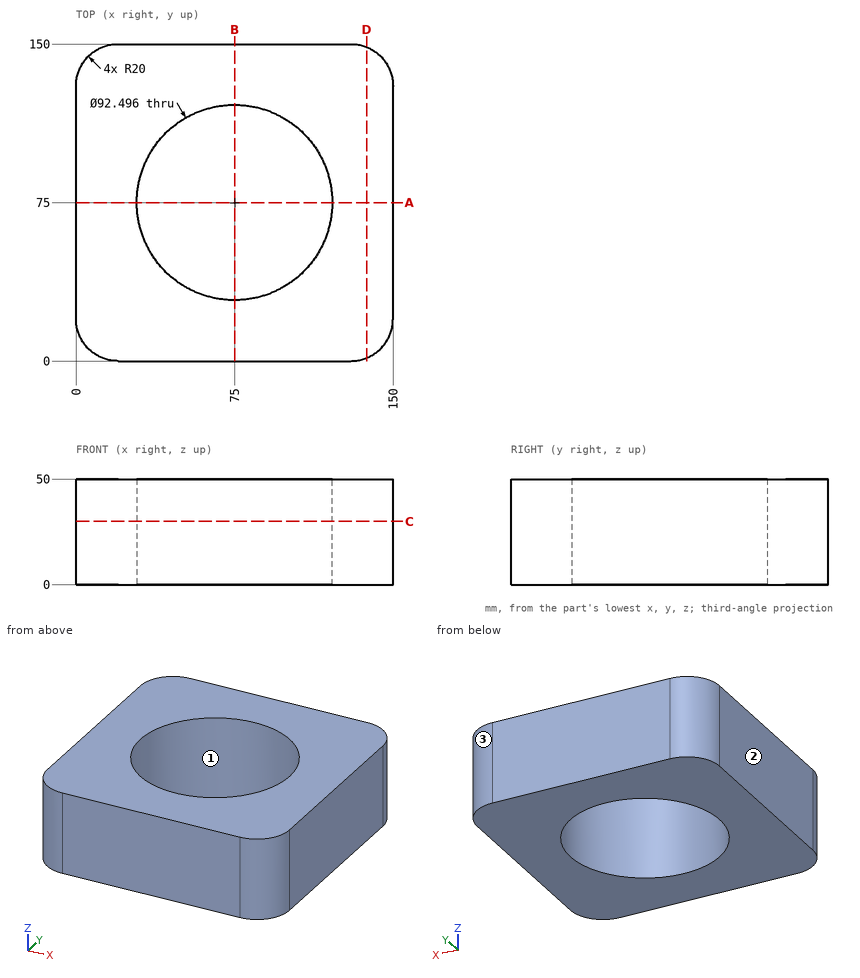
Print and shaded views of the part. All mm, measured from the part's lowest x, y and z. Give positions to 0.01 mm unless a question says otherwise; leave off trailing zeros. Write each loop counter-clockwise with the first axis right and the second up, starting at its lowest first coordinate (ties: lowest second). Pieces come first, ordered by that corner, then holes. Notation, with made-up numbers: (2, -19) -> (20, -19) arc R15 ccw to (20, -4) -> close; hole circle Ø7 at (11.5, 10.25). An arc over 180 degrees is marked (long way). Use CSV: the item, a comma, the result in double quotes. Start each with the question number.
1) Cut at C-C on z = 30. List the corners of the cut face in (x, y), plus the area to 3 significant figures.
2) Drill centre lines: L1, parallel to X at y = 75, z = 38.5; L2, parallel to X at y = 38.5, z = 36.5. Where is each one in solid material? Low to high.
3) Cut at D-D on x = 137.5. List the corners of the cut face in (y, z).
4) Pin check, flat tip, straight feed: P1, Ø5, axis at y = 18, z = 31, coming from the -X side. Stop position of the tip, or through.
5) Cut at A-A on y = 75. List the corners of the cut face in (x, z).
6) Two-plate mould, pull along Y, no slides. Class the marked faces 1, 2 and 3: released by +Y, released by -Y, zero draft, split by the parting line, or undercut.
Final values:
1,outline,"(0, 20) arc R20 ccw to (20, 0) -> (130, 0) arc R20 ccw to (150, 20) -> (150, 130) arc R20 ccw to (130, 150) -> (20, 150) arc R20 ccw to (0, 130) -> close; hole circle Ø92.5 at (75, 75)"
1,area,"15,400 mm2"
2,L1,"x = 0 to 28.75, 121.25 to 150"
2,L2,"x = 0 to 46.6, 103.4 to 150"
3,outline,"(1.46, 0) -> (148.54, 0) -> (148.54, 50) -> (1.46, 50) -> close"
4,P1,"stops at x = 0"
5,outline,"(0, 0) -> (28.75, 0) -> (28.75, 50) -> (0, 50) -> close; (121.25, 0) -> (150, 0) -> (150, 50) -> (121.25, 50) -> close"
6,face 1,"undercut"
6,face 2,"zero draft"
6,face 3,"released by +Y"
